```python
from build123d import *

# Parameters (mm, degrees)
SKETCH1_W           = 30
SKETCH1_H           = 30
BOSS_EXTRUDE1_DEPTH = 3
SKETCH3_R           = 3
BOSS_EXTRUDE2_DEPTH = 6
FILLET2_R           = 1
FILLET3_R           = 2
FILLET4_R           = 2
FILLET5_R           = 2
FILLET6_R           = 2


with BuildPart() as part:
    # Sketch1 → Boss-Extrude1 (new body)
    with BuildSketch(Plane(origin=(0, 0, 0), x_dir=(1, 0, 0), z_dir=(0, 1, 0))):
        with Locations((15, 15)):
            Rectangle(SKETCH1_W, SKETCH1_H)
    extrude(amount=BOSS_EXTRUDE1_DEPTH)

    # Sketch3 → Boss-Extrude2 (add)
    with BuildSketch(Plane(origin=(0, 3, 0), x_dir=(1, 0, 0), z_dir=(0, 1, 0))):
        with Locations(Location((15, 15, 0), (0, 0, 90))):
            Circle(SKETCH3_R)
    extrude(amount=BOSS_EXTRUDE2_DEPTH)

    # Fillet2
    fillet2_edges = [part.edges().sort_by_distance(p)[0] for p in [
        (15, 9, -12),
    ]]
    fillet(fillet2_edges, radius=FILLET2_R)

    # Fillet3
    fillet3_edges = [part.edges().sort_by_distance(p)[0] for p in [
        (15, 0, 0),
        (0, 0, -15),
    ]]
    fillet(fillet3_edges, radius=FILLET3_R)

    # Fillet4
    fillet4_edges = [part.edges().sort_by_distance(p)[0] for p in [
        (30, 0, -16),
        (0.585786438, 0.585786438, -30),
        (30, 0.585786438, -0.585786438),
        (16, 0, -30),
        (0, 2.5, -30),
        (30, 2.5, 0),
    ]]
    fillet(fillet4_edges, radius=FILLET4_R)

    # Fillet5
    # the kernel refuses this fillet: 2 mm, written as the material it takes off along each edge
    with BuildSketch(Plane(origin=(2, 2, -2), x_dir=(-1, 0, 0), z_dir=(0, 0, 1))) as fillet5_piece_1_section:
        Polygon((0, 0), (FILLET5_R, 0), (FILLET5_R, FILLET5_R), (0, FILLET5_R), align=None)
    fillet5_piece_1 = extrude(amount=FILLET5_R, mode=Mode.PRIVATE)
    fillet5_piece_1 = fillet5_piece_1 - Plane(origin=(2, 2, -2), x_dir=(0.7071067811865475, 0.7071067811865475, 0), z_dir=(0, 0, 1)) * Sphere(FILLET5_R, mode=Mode.PRIVATE)
    add(fillet5_piece_1, mode=Mode.SUBTRACT)
    with BuildSketch(Plane(origin=(0, 2, 0), x_dir=(1, 0, 0), z_dir=(0, 1, 0))) as fillet5_piece_2:
        with BuildLine():
            CenterArc((FILLET5_R, FILLET5_R), FILLET5_R, 180, 90)
            Line((0, FILLET5_R), (0, 0))
            Line((0, 0), (FILLET5_R, 0))
        make_face()
    extrude(amount=6, mode=Mode.SUBTRACT)

    # Fillet6
    # the kernel refuses this fillet: 2 mm, written as the material it takes off along each edge
    with BuildSketch(Plane(origin=(28, 2, -28), x_dir=(0, 0, -1), z_dir=(1, 0, 0))) as fillet6_piece_1_section:
        Polygon((0, 0), (FILLET6_R, 0), (FILLET6_R, -FILLET6_R), (0, -FILLET6_R), align=None)
    fillet6_piece_1 = extrude(amount=FILLET6_R, mode=Mode.PRIVATE)
    fillet6_piece_1 = fillet6_piece_1 - Plane(origin=(28, 2, -28), x_dir=(0, 0.7071067811865475, 0.7071067811865475), z_dir=(1, 0, 0)) * Sphere(FILLET6_R, mode=Mode.PRIVATE)
    add(fillet6_piece_1, mode=Mode.SUBTRACT)
    with BuildSketch(Plane(origin=(30, 2, -30), x_dir=(0, 0, 1), z_dir=(0, 1, 0))) as fillet6_piece_2:
        with BuildLine():
            CenterArc((FILLET6_R, -FILLET6_R), FILLET6_R, 90, 90)
            Line((0, -FILLET6_R), (0, 0))
            Line((0, 0), (FILLET6_R, 0))
        make_face()
    extrude(amount=6, mode=Mode.SUBTRACT)


solid = part.part
```
The listing builds one solid part. Answer for the finished solid, in the listing's coordinates (mm). A direction names the side the tool comes from. Round coordinates to 2 decimals unless told otherwise and drop trailing zeros. Loops run counter-clockwise (first coordinate to the right, second up) from the corner with the lowest first, then second, coordinate; pieces in that order, holes last. Notation, with made-up numbers: (48, 42.5) - (88, 42.5) arc R28 cw to (88, 74.5) - close; hole circle Ø2 at (26, -0.5). An arc over 180 degrees is marked (long way). Return JSON: item names as keys, results as strings. Group by question number.
1. The part is cut by section B-B on x = 15. Determine the outline of the cut face in (y, z).
2. The part is cut by section D-D on x = 4. Determine the outline of the cut face in (y, z), then the cut area to 3 significant figures.
3. Each of these flat-tipped pins is pushed along its axis until it touches: P1, Ø1, axis at x = 27, z = -18, coming from the +Y side; P2, Ø1.5, axis at y = 6, z = -17.5, coming from the +X side; P3, Ø3, axis at y = 7, z = -16.5, coming from the +X side. Where does it stop, or does it pass through?
4. Which of the six approach directions +Z, -Z, +X, -X, +Y, -Y give full straight-line access (tool end or side, diameter ignored) to faces 1 (the cylindrical face through (29.43, 2.49, -29.4)), 2 (the cylindrical face through (17.93, 5.46, -14.35))?
5. The part is cut by section C-C on y = 1. Determine the outline of the cut face in (x, z).
6. Consider probe 1 along Y at (x, z) = (25.25, -17.25); probe 2 along Z at (x, y) = (16.5, 4.25); probe 3 along Z at (x, y) = (24.5, 0.5). Determine where each line is inside the solid, lowest interval first.
7. The part is cut by section A-A on z = -15. Determine the outline of the cut face in (x, y).
Resolved:
{
 "1": {"outline": "(0, -28) arc R2 ccw to (2, -30) - (3, -30) - (3, -18) - (8, -18) arc R1 ccw to (9, -17) - (9, -13) arc R1 ccw to (8, -12) - (3, -12) - (3, 0) - (2, 0) arc R2 ccw to (0, -2) - close"},
 "2": {"outline": "(0, -28) arc R2 ccw to (2, -30) - (3, -30) - (3, 0) - (2, 0) arc R2 ccw to (0, -2) - close", "area": "88.3 mm²"},
 "3": {"P1": "stops at y = 3", "P2": "stops at x = 17.44", "P3": "stops at x = 18"},
 "4": {"face 1": "-Z, +X, +Y, -Y", "face 2": "+Y"},
 "5": {"outline": "(0.27, -28) arc R1.73 ccw to (2, -29.73) - (28, -29.73) arc R1.73 ccw to (29.73, -28) - (29.73, -2) arc R1.73 ccw to (28, -0.27) - (2, -0.27) arc R1.73 ccw to (0.27, -2) - close"},
 "6": {"probe 1": "y = 0 to 3", "probe 2": "z = -17.6 to -12.4", "probe 3": "z = -29.32 to -0.68"},
 "7": {"outline": "(0, 2) arc R2 ccw to (2, 0) - (28, 0) arc R2 ccw to (30, 2) - (30, 3) - (18, 3) - (18, 8) arc R1 ccw to (17, 9) - (13, 9) arc R1 ccw to (12, 8) - (12, 3) - (0, 3) - close"}
}
